Source: CAD feature listing. Evaluate the final solid. Frame: model axes, mm. Face numbers are marked on the shaded views. A direction names the side the tool comes from. Coordinates: 2 decimals unless noted, no trailing zeros. Loops run counter-clockwise (first coordinate to the right, second up) from the corner with the lowest first, then second, coordinate; pieces in that order, holes last.
Item 1: Pin query (flat end, axial travel): pin 1 Ø6 at (x, z) = (134.5, -148.5) entering from -Y; pin 2 Ø2 at (x, z) = (23.5, -52.5) entering from -Y; pin 3 Ø5 at (x, z) = (151.62, -164.52) entering from +Y; pin 4 Ø12 at (x, z) = (143, -36.5) entering from -Y. Return the tip coordinate at first contact, or that it passes through.
Item 2: Section query C-C, the plane z = -106. Return the cut outline in (x, y).
Item 3: Reachability of the marked faces 4 and 5 from +Z, -Z, +X, -X, +Y, -Y: full face, straight path, thin tool, end or side. Return the list, or none.
Item 4: Section query B-B, the plane z = -30. Return the cut outline in (x, y).
Item 5: Line query: probe 1 along Z at (x, y) = (35, -166); probe 2 along X at (y, z) = (-94, -131.5); probe 3 along X at (y, z) = (-28, -40). Output: solid intervals per line, ascending.
Item 6: Pull-direction query (X, two-part tool) for the marked faces 1, 2 and 3; classes: +X half, -X half, draft (parallel to the pull), parting line (faces both ways), or undercut.
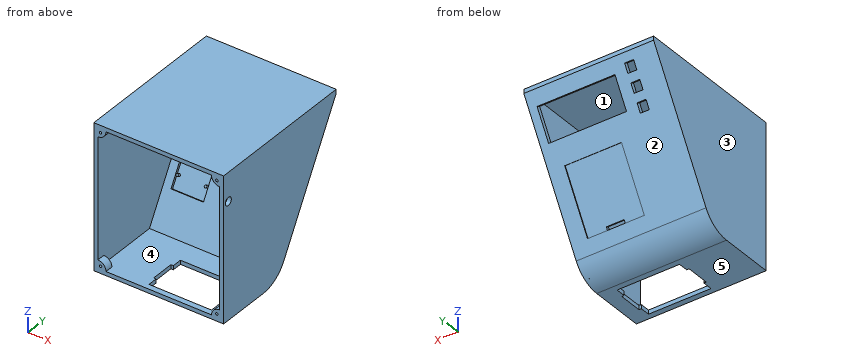
```python
from build123d import *

# Parameters (mm, degrees)
BOSS_EXTRUDE1_DEPTH  = 5
SKETCH2_W            = 160
SKETCH2_H            = 200
BOSS_EXTRUDE2_DEPTH  = 5
SKETCH4_W            = 160
SKETCH4_H            = 190
BOSS_EXTRUDE4_DEPTH  = 5
SKETCH5_W            = 160
SKETCH5_H            = 90
BOSS_EXTRUDE5_DEPTH  = 5
SKETCH6_W            = 96
SKETCH6_H            = 39
SKETCH6_W_2          = 11
SKETCH6_H_2          = 11
CUT_EXTRUDE2_DEPTH   = 5
FILLET1_R            = 40
SKETCH7_W            = 70
SKETCH7_H            = 77
CUT_EXTRUDE3_DEPTH   = 1
SKETCH8_W            = 22
SKETCH8_H            = 4
CUT_EXTRUDE4_DEPTH   = 4
SKETCH9_W            = 40
SKETCH9_H            = 60
CUT_EXTRUDE5_DEPTH   = 5
SKETCH12_W           = 40
SKETCH12_H           = 60
BOSS_EXTRUDE6_DEPTH  = 2
SKETCH14_W           = 77
SKETCH14_H           = 53
CUT_EXTRUDE6_DEPTH   = 5
SKETCH15_W           = 3
SKETCH15_H           = 29
CUT_EXTRUDE7_DEPTH   = 5
SKETCH17_R           = 1.75
CUT_EXTRUDE9_DEPTH   = 4
SKETCH21_R           = 1.5
BOSS_EXTRUDE8_DEPTH  = 4
SKETCH23_R           = 1.5
BOSS_EXTRUDE9_DEPTH  = 10
SKETCH25_R           = 1.5
BOSS_EXTRUDE10_DEPTH = 10
SKETCH33_R           = 5
CUT_EXTRUDE14_DEPTH  = 10


with BuildPart() as part:
    # Sketch1 → Boss-Extrude1 (new body)
    with BuildSketch(Plane(origin=(0, 0, 0), x_dir=(0, 0, -1), z_dir=(1, 0, 0))):
        Polygon((0, 0), (173.205080757, -100), (173.205080757, -190), (0, -190), align=None)
    boss_extrude1 = extrude(amount=BOSS_EXTRUDE1_DEPTH)

    # Sketch2 → Boss-Extrude2 (add)
    with BuildSketch(Plane(origin=(0, 0, 0), x_dir=(1, 0, 0), z_dir=(0, 0.8660254037844382, -0.5000000000000011))):
        with Locations((80, 100)):
            Rectangle(SKETCH2_W, SKETCH2_H)
    extrude(amount=-BOSS_EXTRUDE2_DEPTH)

    # Sketch4 → Boss-Extrude4 (add)
    with BuildSketch(Plane.XY):
        with Locations((80, -95)):
            Rectangle(SKETCH4_W, SKETCH4_H)
    extrude(amount=BOSS_EXTRUDE4_DEPTH)

    # Sketch5 → Boss-Extrude5 (add)
    with BuildSketch(Plane(origin=(0, 0, -173.205080757), x_dir=(-1, 0, 0), z_dir=(0, 0, -1))):
        with Locations((-80, -145)):
            Rectangle(SKETCH5_W, SKETCH5_H)
    extrude(amount=-BOSS_EXTRUDE5_DEPTH)

    # Mirror1: Boss-Extrude1 across plane
    add(boss_extrude1.mirror(Plane.ZY.offset(-80)))

    # Sketch6 → Cut-Extrude2 (cut)
    with BuildSketch(Plane(origin=(0, 0, 0), x_dir=(1, 0, 0), z_dir=(0, 0.8660254037844382, -0.5000000000000011))):
        with Locations((102, 36.815172727)):
            Rectangle(SKETCH6_W, SKETCH6_H)
        with Locations((34, 15.815172727)):
            Rectangle(SKETCH6_W_2, SKETCH6_H_2)
        with Locations((34, 36.815172727)):
            Rectangle(SKETCH6_W_2, SKETCH6_H_2)
        with Locations((34, 57.815172727)):
            Rectangle(SKETCH6_W_2, SKETCH6_H_2)
    extrude(amount=-CUT_EXTRUDE2_DEPTH, mode=Mode.SUBTRACT)

    # Fillet1
    fillet1_edges = [part.edges().sort_by_distance(p)[0] for p in [
        (80, -100, -173.205080757),
    ]]
    fillet(fillet1_edges, radius=FILLET1_R)

    # Sketch7 → Cut-Extrude3 (cut)
    with BuildSketch(Plane(origin=(0, 0, 0), x_dir=(1, 0, 0), z_dir=(0, 0.8660254037844382, -0.5000000000000011))):
        with Locations((105, 121.815172727)):
            Rectangle(SKETCH7_W, SKETCH7_H)
    extrude(amount=-CUT_EXTRUDE3_DEPTH, mode=Mode.SUBTRACT)

    # Sketch8 → Cut-Extrude4 (cut)
    with BuildSketch(Plane(origin=(0, -0.866025403784426, 0.4999999999999943), x_dir=(1, 0, 0), z_dir=(0, 0.8660254037844382, -0.5000000000000011))):
        with Locations((105, 158.315172727)):
            Rectangle(SKETCH8_W, SKETCH8_H)
    extrude(amount=-CUT_EXTRUDE4_DEPTH, mode=Mode.SUBTRACT)

    # Sketch9 → Cut-Extrude5 (cut)
    with BuildSketch(Plane(origin=(0, 0, 0), x_dir=(1, 0, 0), z_dir=(0, 0.8660254037844382, -0.5000000000000011))):
        with Locations((35, 121.815172727)):
            Rectangle(SKETCH9_W, SKETCH9_H)
    extrude(amount=-CUT_EXTRUDE5_DEPTH, mode=Mode.SUBTRACT)

    # Sketch12 → Boss-Extrude6 (add)
    with BuildSketch(Plane(origin=(0, 0, 0), x_dir=(1, 0, 0), z_dir=(0, 0.8660254037844382, -0.5000000000000011))):
        with Locations((35, 121.815172727)):
            Rectangle(SKETCH12_W, SKETCH12_H)
    extrude(amount=-BOSS_EXTRUDE6_DEPTH)

    # Sketch14 → Cut-Extrude6 (cut)
    with BuildSketch(Plane(origin=(0, 0, -173.205080757), x_dir=(-1, 0, 0), z_dir=(0, 0, -1))):
        with Locations((-101.5, -156.594010768)):
            Rectangle(SKETCH14_W, SKETCH14_H)
    extrude(amount=-CUT_EXTRUDE6_DEPTH, mode=Mode.SUBTRACT)

    # Sketch15 → Cut-Extrude7 (cut)
    with BuildSketch(Plane(origin=(0, 0, -173.205080757), x_dir=(-1, 0, 0), z_dir=(0, 0, -1))):
        with Locations((-61.5, -156.594010768)):
            Rectangle(SKETCH15_W, SKETCH15_H)
        with Locations((-141.5, -156.594010768)):
            Rectangle(SKETCH15_W, SKETCH15_H)
    extrude(amount=-CUT_EXTRUDE7_DEPTH, mode=Mode.SUBTRACT)

    # Sketch17 → Cut-Extrude9 (cut)
    with BuildSketch(Plane(origin=(0, -4.330127019, 2.5), x_dir=(-1, 0, 0), z_dir=(0, -0.8660254037844382, 0.500000000000001))):
        with Locations(Location((-54.75, 64.989476433, 0), (0, 0, 90))):
            Circle(SKETCH17_R)
        with Locations(Location((-149.25, 64.989476433, 0), (0, 0, 270))):
            Circle(SKETCH17_R)
        with Locations(Location((-54.75, 8.489476433, 0), (0, 0, 270))):
            Circle(SKETCH17_R)
        with Locations(Location((-149.25, 8.489476433, 0), (0, 0, 90))):
            Circle(SKETCH17_R)
    extrude(amount=-CUT_EXTRUDE9_DEPTH, mode=Mode.SUBTRACT)

    # Sketch21 → Boss-Extrude8 (add)
    with BuildSketch(Plane(origin=(0, -1.732050808, 1), x_dir=(-1, 0, 0), z_dir=(0, -0.8660254037844382, 0.500000000000001))):
        with Locations(Location((-48.5, 98.315172727, 0), (0, 0, 270))):
            Circle(SKETCH21_R)
        with Locations(Location((-21.5, 97.315172727, 0), (0, 0, 270))):
            Circle(SKETCH21_R)
        with Locations(Location((-17.5, 136.315172727, 0), (0, 0, 270))):
            Circle(SKETCH21_R)
        with Locations(Location((-52.5, 136.315172727, 0), (0, 0, 270))):
            Circle(SKETCH21_R)
    extrude(amount=BOSS_EXTRUDE8_DEPTH)

    # Sketch23 → Boss-Extrude9 (add)
    with BuildSketch(Plane(origin=(0, -190, 0), x_dir=(-1, 0, 0), z_dir=(0, -1, 0))):
        with BuildLine():
            Line((-155, 0), (-145, 0))
            ThreePointArc((-145, 0), (-147.928932188, 7.071067812), (-155, 10))
            Line((-155, 10), (-155, 0))
        make_face()
        with Locations(Location((-151.751738587, 3.801157428, 0), (0, 0, 90))):
            Circle(SKETCH23_R, mode=Mode.SUBTRACT)
    boss_extrude9 = extrude(amount=-BOSS_EXTRUDE9_DEPTH)

    # Mirror2: Boss-Extrude9 across plane
    add(boss_extrude9.mirror(Plane.ZY.offset(-80)))

    # Sketch25 → Boss-Extrude10 (add)
    with BuildSketch(Plane(origin=(0, -190, 0), x_dir=(-1, 0, 0), z_dir=(0, -1, 0))):
        with BuildLine():
            Line((-155, 168.205080757), (-145, 168.205080757))
            ThreePointArc((-145, 168.205080757), (-147.928932188, 161.134012945), (-155, 158.205080757))
            Line((-155, 158.205080757), (-155, 168.205080757))
        make_face()
        with Locations(Location((-151.620258089, 164.520335906, 0), (0, 0, 90))):
            Circle(SKETCH25_R, mode=Mode.SUBTRACT)
    boss_extrude10 = extrude(amount=-BOSS_EXTRUDE10_DEPTH)

    # Mirror4: Boss-Extrude10 across plane
    add(boss_extrude10.mirror(Plane.ZY.offset(-80)))

    # Sketch33 → Cut-Extrude14 (cut)
    with BuildSketch(Plane(origin=(160, 0, 0), x_dir=(0, 0, -1), z_dir=(1, 0, 0))):
        with Locations((30, -182)):
            Circle(SKETCH33_R)
    extrude(amount=-CUT_EXTRUDE14_DEPTH, mode=Mode.SUBTRACT)


solid = part.part
```
Verdict:
1. pin 1: stops at y = -93.24
1. pin 2: stops at y = -36.66
1. pin 3: stops at y = -95.35
1. pin 4: passes through
2. outline: (0, -190) - (5, -190) - (5, -66.97) - (15, -66.97) - (15, -63.51) - (55, -63.51) - (55, -66.97) - (155, -66.97) - (155, -190) - (160, -190) - (160, -61.2) - (140, -61.2) - (140, -62.35) - (70, -62.35) - (70, -61.2) - (0, -61.2) - close
3. face 4: none
3. face 5: -Z, +X, -X, +Y, -Y
4. outline: (0, -190) - (5, -190) - (5, -23.09) - (28.5, -23.09) - (28.5, -17.32) - (0, -17.32) - close; (39.5, -23.09) - (54, -23.09) - (54, -17.32) - (39.5, -17.32) - close; (150, -23.09) - (155, -23.09) - (155, -177) - (160, -177) - (160, -17.32) - (150, -17.32) - close; (155, -190) - (160, -190) - (160, -187) - (155, -187) - close
5. probe 1: z = -173.21 to -168.21, 0 to 5
5. probe 2: x = 0 to 5, 155 to 160
5. probe 3: x = 0 to 54, 150 to 160
6. face 1: undercut
6. face 2: draft
6. face 3: -X half
